Work out the finished part from the listing and answer in its coordinate system (mm). A direction names the side the tool comes from. Coordinates: 2 decimals unless noted, no trailing zeros. Loops run counter-clockwise (first coordinate to the right, second up) from the corner with the lowest first, then second, coordinate; pieces in that order, holes last. Notation, with made-up numbers: (12.25, 22.5) -> (52.25, 22.5) arc R22 ccw to (52.25, 60.5) -> close; hole circle Ø8 at (43.5, -27). An arc over 180 degrees is marked (long way). One line per question, with ' | ' between items.
```python
from build123d import *

# Parameters (mm, degrees)
SALIENTE_EXTRUIR1_DEPTH = 2743.2


with BuildPart() as part:
    # Croquis1 → Saliente-Extruir1 (new body)
    with BuildSketch(Plane.XY):
        Polygon((-139.7, -174.625), (-139.7, -180.975), (-184.15, -180.975), (-184.15, -215.9), (31.75, -215.9), (31.75, -57.15), (-6.35, -57.15), (-6.35, 0), (0, 0), (0, -50.8), (38.1, -50.8), (38.1, -222.25), (-190.5, -222.25), (-190.5, -174.625), align=None)
    extrude(amount=-SALIENTE_EXTRUIR1_DEPTH)


solid = part.part
```
1) The mould has two halves that part along Y. Classify faces 4 (the face through (0, -25, -1352)), 5 (the face through (-165, -174.625, -1352)), 6 (the face through (31.75, -138, -1352)): released by +Y, released by -Y, zero draft, split by the parting line, or undercut.
Check values:
face 4: zero draft | face 5: released by +Y | face 6: undercut
2) Find section B-B (x = -47). Write down the section's boundary in (y, z).
Check values:
outline: (-222.25, -2743.2) -> (-215.9, -2743.2) -> (-215.9, 0) -> (-222.25, 0) -> close
3) Find section C-C (y = -128). Write down the section's boundary in (x, z).
Check values:
outline: (31.75, -2743.2) -> (38.1, -2743.2) -> (38.1, 0) -> (31.75, 0) -> close
4) For faces 1 (the face through (-6.35, -29, -1352)), 2 (the face through (-190.5, -199, -1352)), 3 (the face through (-162, -180.975, -1352)), determine the directions among +Z, -Z, +X, -X, +Y, -Y from which every point of the face is accessible in a straight line to the end or side of a thin tool.
Check values:
face 1: +Z, -Z, -X, +Y | face 2: +Z, -Z, -X, +Y, -Y | face 3: +Z, -Z
5) Find the intervals of material crossed by line 1 along Y through (x, z) = (-163, -2385) (3 decimals); line 2 along X through (y, z) = (-195.5, -2458); line 3 along Y through (x, z) = (23, -501.5), in increasing order.
Check values:
line 1: y = -222.25 to -215.9, -180.975 to -174.625 | line 2: x = -190.5 to -184.15, 31.75 to 38.1 | line 3: y = -222.25 to -215.9, -57.15 to -50.8
6) Flat-ended cylindrical pins translate along their axes: pin 1 (4 mm diameter, centred on x = -63.5, z = -1632.5, fed in from +Y); pin 2 (2 mm diameter, centred on y = -170, z = -512, fed in from -X); pin 3 (11.5 mm diameter, centred on x = 21.5, z = -1097, fed in from +Y). Find the tip coordinate at first contact, or state that the pin passes through.
Check values:
pin 1: stops at y = -215.9 | pin 2: stops at x = 31.75 | pin 3: stops at y = -50.8
7) Find section A-A (z = -2448). Write down the section's boundary in (x, y) (3 decimals).
Check values:
outline: (-190.5, -222.25) -> (38.1, -222.25) -> (38.1, -50.8) -> (0, -50.8) -> (0, 0) -> (-6.35, 0) -> (-6.35, -57.15) -> (31.75, -57.15) -> (31.75, -215.9) -> (-184.15, -215.9) -> (-184.15, -180.975) -> (-139.7, -180.975) -> (-139.7, -174.625) -> (-190.5, -174.625) -> close
